Read the model definition and answer for the solid it produces. Units are mm, in the model's axes. Face numbers are marked on the shaded views. A direction names the side the tool comes from. Round coordinates to 2 decimals unless told otherwise and drop trailing zeros. Write each loop counter-clockwise with the first axis right and the second up, starting at its lowest first coordinate (ties: lowest second). Pieces come first, ordered by that corner, then holes. Notation, with made-up numbers: (12, -21.5) -> (60, -21.5) arc R13 ccw to (60, -15.5) -> close; hole circle Ø2 at (32, 7.5). An arc over 180 degrees is marked (long way). Return JSON: item names as keys, results as strings.
from build123d import *

# Parameters (mm, degrees)
SKETCH1_W           = 10.24
SKETCH1_H           = 10.24
BOSS_EXTRUDE1_DEPTH = 0.54
SKETCH2_W           = 9.65
SKETCH2_H           = 6.88
BOSS_EXTRUDE2_DEPTH = 2.46
FILLET1_R           = 0.5
SKETCH3_R           = 0.5
CUT_EXTRUDE1_DEPTH  = 0.1
CUT_EXTRUDE2_DEPTH  = 0.1


with BuildPart() as part:
    # Sketch1 → Boss-Extrude1 (new body)
    with BuildSketch(Plane(origin=(0, 0, 0), x_dir=(1, 0, 0), z_dir=(0, 1, 0))):
        Rectangle(SKETCH1_W, SKETCH1_H)
    extrude(amount=BOSS_EXTRUDE1_DEPTH)

    # Sketch2 → Boss-Extrude2 (add)
    with BuildSketch(Plane(origin=(0, 0.54, 0), x_dir=(1, 0, 0), z_dir=(0, 1, 0))):
        Rectangle(SKETCH2_W, SKETCH2_H)
    extrude(amount=BOSS_EXTRUDE2_DEPTH)

    # Fillet1
    fillet1_edges = [part.edges().sort_by_distance(p)[0] for p in [
        (4.825, 1.77, 3.44),
        (4.825, 1.77, -3.44),
        (-4.825, 1.77, -3.44),
        (-4.825, 1.77, 3.44),
    ]]
    fillet(fillet1_edges, radius=FILLET1_R)

    # Sketch3 → Cut-Extrude1 (cut)
    with BuildSketch(Plane(origin=(0, 3, 0), x_dir=(1, 0, 0), z_dir=(0, 1, 0))):
        with Locations((-3.825, -2.44)):
            Circle(SKETCH3_R)
    extrude(amount=-CUT_EXTRUDE1_DEPTH, mode=Mode.SUBTRACT)

    # Sketch4 → Cut-Extrude2 (cut)
    with BuildSketch(Plane(origin=(0, 3, 0), x_dir=(1, 0, 0), z_dir=(0, 1, 0))):
        Polygon((-4.208905933, 1.144195858), (-3.716714341, 2.685187069), (-3.560676473, 2.685187069), (-3.06817218, 1.144195858), (-3.234529186, 1.144195858), (-3.369303376, 1.604491934), (-3.907774737, 1.604491934), (-4.042236227, 1.144195858), align=None)
        with BuildLine():
            Line((-3.855240946, 1.78460779), (-3.422149869, 1.78460779))
            Line((-3.422149869, 1.78460779), (-3.550982738, 2.208005131))
            add(Edge.make_bspline(
                [(-3.550982738, 2.208005131), (-3.555802408, 2.22384126), (-3.565212111, 2.254758994), (-3.578537108, 2.300032071), (-3.591326078, 2.342972738), (-3.602250322, 2.38388053), (-3.61311318, 2.422223196), (-3.622481656, 2.458427427), (-3.630891424, 2.492313544), (-3.636057432, 2.514238953), (-3.638539057, 2.524771385)],
                knots=[0, 0, 0, 0, 4.9659e-05, 9.6953e-05, 0.000141582, 0.000184064, 0.000223969, 0.000261133, 0.000296247, 0.00032871, 0.00032871, 0.00032871, 0.00032871], degree=3))
            add(Edge.make_bspline(
                [(-3.638539057, 2.524771385), (-3.643044276, 2.500238484), (-3.65204873, 2.451205272), (-3.668927225, 2.378161214), (-3.687705063, 2.305248967), (-3.702651529, 2.257146174), (-3.710147617, 2.233021222)],
                knots=[0, 0, 0, 0, 7.482e-05, 0.00014954, 0.000224855, 0.000300632, 0.000300632, 0.000300632, 0.000300632], degree=3))
            Line((-3.710147617, 2.233021222), (-3.855240946, 1.78460779))
        make_face(mode=Mode.SUBTRACT)
        with BuildLine():
            Line((-2.888056324, 1.144195858), (-2.888056324, 2.685187069))
            Line((-2.888056324, 2.685187069), (-2.413375996, 2.685187069))
            add(Edge.make_bspline(
                [(-2.413375996, 2.685187069), (-2.399822743, 2.685199787), (-2.373748311, 2.685224254), (-2.336020957, 2.683378466), (-2.30094543, 2.681513344), (-2.268644767, 2.677914478), (-2.239094529, 2.673984648), (-2.212324896, 2.66907385), (-2.188330523, 2.662867435), (-2.173405243, 2.657853313), (-2.166342096, 2.655480461)],
                knots=[0, 0, 0, 0, 4.0652e-05, 7.8209e-05, 0.0001133, 0.000146002, 0.000175676, 0.000202722, 0.000227599, 0.000249948, 0.000249948, 0.000249948, 0.000249948], degree=3))
            add(Edge.make_bspline(
                [(-2.166342096, 2.655480461), (-2.15739835, 2.652018743), (-2.139532052, 2.645103513), (-2.114366349, 2.631451435), (-2.09035999, 2.616070999), (-2.067785044, 2.598561502), (-2.046773915, 2.578653074), (-2.026997713, 2.556783142), (-2.008849339, 2.532502116), (-1.992128119, 2.506327155), (-1.976558078, 2.478522333), (-1.963702465, 2.448747644), (-1.952154302, 2.417630839), (-1.943367912, 2.384807465), (-1.935942576, 2.3505097), (-1.931213224, 2.314633597), (-1.927842425, 2.277176403), (-1.92757514, 2.251687241), (-1.927438426, 2.238649843)],
                knots=[0, 0, 0, 0, 2.8745e-05, 5.7421e-05, 8.5698e-05, 0.000114221, 0.000142979, 0.000172428, 0.000202572, 0.000233798, 0.000265568, 0.000298048, 0.000330989, 0.000365052, 0.000399887, 0.000436194, 0.000473536, 0.000512635, 0.000512635, 0.000512635, 0.000512635], degree=3))
            add(Edge.make_bspline(
                [(-1.927438426, 2.238649843), (-1.927703132, 2.221543206), (-1.928220835, 2.188086636), (-1.93330388, 2.139152317), (-1.941751736, 2.092755631), (-1.953277936, 2.048673687), (-1.968247434, 2.006973056), (-1.986783863, 1.967763319), (-2.008529273, 1.930904056), (-2.033354788, 1.89632649), (-2.062609276, 1.864852564), (-2.097135287, 1.83792685), (-2.136198408, 1.814898294), (-2.180286283, 1.796594194), (-2.228949187, 1.781809429), (-2.282628295, 1.771730453), (-2.3411162, 1.765892858), (-2.381674975, 1.765038653), (-2.402744157, 1.764594917)],
                knots=[0, 0, 0, 0, 5.1307e-05, 0.000100344, 0.000147388, 0.000192669, 0.000236884, 0.000280107, 0.000322581, 0.000365113, 0.000407588, 0.000451004, 0.000495999, 0.000543218, 0.000593866, 0.000648324, 0.000706789, 0.000769993, 0.000769993, 0.000769993, 0.000769993], degree=3))
            Line((-2.402744157, 1.764594917), (-2.727953341, 1.764594917))
            Line((-2.727953341, 1.764594917), (-2.727953341, 1.144195858))
            Line((-2.727953341, 1.144195858), (-2.888056324, 1.144195858))
        make_face()
        with BuildLine():
            Line((-2.727953341, 1.944710773), (-2.392737721, 1.944710773))
            add(Edge.make_bspline(
                [(-2.392737721, 1.944710773), (-2.380016461, 1.944996579), (-2.355368886, 1.945550331), (-2.319593959, 1.948503929), (-2.28645598, 1.954137106), (-2.255965679, 1.961851391), (-2.228207938, 1.971910844), (-2.203044284, 1.984006949), (-2.180618389, 1.998565987), (-2.160576979, 2.015206906), (-2.143495605, 2.034541806), (-2.128130148, 2.05560326), (-2.115669137, 2.079385756), (-2.105485872, 2.105324963), (-2.097214244, 2.133336313), (-2.091756565, 2.163637248), (-2.08826807, 2.196145263), (-2.087788442, 2.21862743), (-2.087541409, 2.230206912)],
                knots=[0, 0, 0, 0, 3.817e-05, 7.3955e-05, 0.000107576, 0.000138899, 0.000168179, 0.00019601, 0.000222464, 0.000248208, 0.000273892, 0.000299664, 0.000326244, 0.000354174, 0.000383168, 0.000413711, 0.000446413, 0.000481145, 0.000481145, 0.000481145, 0.000481145], degree=3))
            add(Edge.make_bspline(
                [(-2.087541409, 2.230206912), (-2.08789706, 2.245247803), (-2.088585266, 2.274352792), (-2.095703866, 2.316217414), (-2.106715605, 2.354836551), (-2.122831996, 2.389433378), (-2.141679929, 2.419771411), (-2.162318289, 2.445723404), (-2.185368747, 2.466112503), (-2.206821105, 2.478820504), (-2.225660971, 2.486835174), (-2.242449858, 2.491781091), (-2.261836205, 2.495665981), (-2.283750042, 2.499067941), (-2.30814868, 2.501936461), (-2.335078678, 2.50362652), (-2.364580349, 2.505013397), (-2.385126647, 2.505051368), (-2.395864732, 2.505071213)],
                knots=[0, 0, 0, 0, 4.5082e-05, 8.7237e-05, 0.000127012, 0.000165211, 0.000201307, 0.000233979, 0.000264337, 0.000293082, 0.000308356, 0.000325668, 0.000345477, 0.000367635, 0.000392187, 0.000419145, 0.000448566, 0.000480775, 0.000480775, 0.000480775, 0.000480775], degree=3))
            Line((-2.395864732, 2.505071213), (-2.727953341, 2.505071213))
            Line((-2.727953341, 2.505071213), (-2.727953341, 1.944710773))
        make_face(mode=Mode.SUBTRACT)
        Polygon((-1.707296825, 1.144195858), (-1.707296825, 2.685187069), (-0.786704673, 2.685187069), (-0.786704673, 2.505071213), (-1.547193842, 2.505071213), (-1.547193842, 2.024762264), (-0.826730419, 2.024762264), (-0.826730419, 1.844646408), (-1.547193842, 1.844646408), (-1.547193842, 1.324311714), (-0.7666918, 1.324311714), (-0.7666918, 1.144195858), align=None)
        with BuildLine():
            Line((-0.646614563, 1.144195858), (-0.157549982, 1.947837784))
            Line((-0.157549982, 1.947837784), (-0.606588817, 2.685187069))
            Line((-0.606588817, 2.685187069), (-0.423658651, 2.685187069))
            Line((-0.423658651, 2.685187069), (-0.181315269, 2.28743122))
            add(Edge.make_bspline(
                [(-0.181315269, 2.28743122), (-0.169736699, 2.268361701), (-0.148036169, 2.232621651), (-0.117649456, 2.182287392), (-0.091062059, 2.139057874), (-0.074879604, 2.112326527), (-0.067492054, 2.100123238)],
                knots=[0, 0, 0, 0, 6.6928e-05, 0.000125437, 0.000176385, 0.000219181, 0.000219181, 0.000219181, 0.000219181], degree=3))
            add(Edge.make_bspline(
                [(-0.067492054, 2.100123238), (-0.049678986, 2.127999568), (-0.012690335, 2.185884479), (0.02309097, 2.244523598), (0.041640643, 2.274923175)],
                knots=[0, 0, 0, 0, 9.9242e-05, 0.000206075, 0.000206075, 0.000206075, 0.000206075], degree=3))
            Line((0.041640643, 2.274923175), (0.291176152, 2.685187069))
            Line((0.291176152, 2.685187069), (0.474106318, 2.685187069))
            Line((0.474106318, 2.685187069), (0.025067483, 1.947212382))
            Line((0.025067483, 1.947212382), (0.514132064, 1.144195858))
            Line((0.514132064, 1.144195858), (0.331201898, 1.144195858))
            Line((0.331201898, 1.144195858), (-0.009642343, 1.703618195))
            add(Edge.make_bspline(
                [(-0.009642343, 1.703618195), (-0.01890825, 1.719051357), (-0.037706972, 1.750362242), (-0.056640217, 1.781591969), (-0.06624125, 1.797428536)],
                knots=[0, 0, 0, 0, 5.4003e-05, 0.000109562, 0.000109562, 0.000109562, 0.000109562], degree=3))
            add(Edge.make_bspline(
                [(-0.06624125, 1.797428536), (-0.074099113, 1.784632259), (-0.088514391, 1.761157446), (-0.107567841, 1.72889146), (-0.123536239, 1.703682546), (-0.132254181, 1.688732713), (-0.135973603, 1.682354517)],
                knots=[0, 0, 0, 0, 4.5049e-05, 8.2642e-05, 0.000112407, 0.000134556, 0.000134556, 0.000134556, 0.000134556], degree=3))
            Line((-0.135973603, 1.682354517), (-0.463684397, 1.144195858))
            Line((-0.463684397, 1.144195858), (-0.646614563, 1.144195858))
        make_face()
    extrude(amount=-CUT_EXTRUDE2_DEPTH, mode=Mode.SUBTRACT)


solid = part.part
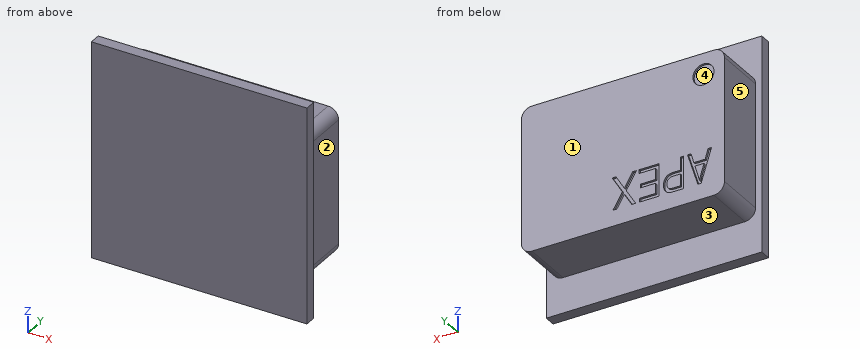
Item 1: Section C-C (z = 2.44) is taken. Give the vertices of the cut face in (x, y) (3 decimals), then the cut area to 3 significant figures.
Worked answers:
{"outline": "(-5.12, 0) -> (5.12, 0) -> (5.12, 0.54) -> (4.825, 0.54) -> (4.825, 3) -> (-3.325, 3) -> (-3.325, 2.9) -> (-4.325, 2.9) -> (-4.325, 3) -> (-4.825, 3) -> (-4.825, 0.54) -> (-5.12, 0.54) -> close", "area": "29.2 mm2"}
Item 2: For a pull along Z with two mould halves and no side action, classify the marked faces 3, 4 and 5 as released by +Z, released by -Z, zero draft, split by the parting line, or undercut.
Worked answers:
{"face 3": "released by -Z", "face 4": "undercut", "face 5": "zero draft"}
Item 3: A tool of negligible diameter and unlimited length cuts with its end or side. For the marked faces 1 and 2, from which of +Z, -Z, +X, -X, +Y, -Y can it reach the whole face along a straight path? Write none if from no direction.
Worked answers:
{"face 1": "+Z, -Z, +X, -X, +Y", "face 2": "+Z, -Z, +X, +Y"}
Item 4: Section A-A (x = 4) is taken. Give the vertices of the cut face in (y, z), then the cut area to 3 significant figures.
Worked answers:
{"outline": "(0, -5.12) -> (0.54, -5.12) -> (0.54, -3.44) -> (3, -3.44) -> (3, 3.44) -> (0.54, 3.44) -> (0.54, 5.12) -> (0, 5.12) -> close", "area": "22.5 mm2"}
Item 5: Straight lines are drawn through the part: L1, parallel to Z at x = 1.25, y = 1.6; L2, parallel to X at y = 0.7, z = 3; L3, parallel to Y at x = -3.25, z = 4.25. For each, find the intervals that lie inside material, in ascending order. Write a range as [from, to].
Worked answers:
{"L1": "z = [-3.44, 3.44]", "L2": "x = [-4.82, 4.82]", "L3": "y = [0, 0.54]"}
Item 6: Section B-B (y = 2.5) is taken. Give the vertices of the cut face in (x, z) (3 decimals), then the cut area to 3 significant figures.
Worked answers:
{"outline": "(-4.825, -2.94) arc R0.5 ccw to (-4.325, -3.44) -> (4.325, -3.44) arc R0.5 ccw to (4.825, -2.94) -> (4.825, 2.94) arc R0.5 ccw to (4.325, 3.44) -> (-4.325, 3.44) arc R0.5 ccw to (-4.825, 2.94) -> close", "area": "66.2 mm2"}
